```python
from build123d import *

# Parameters (mm, degrees)
SKETCH1_W              = 55.88
SKETCH1_H              = 63.5
EXTRUDE1_DEPTH         = 25.4
EXTRUDE1_DEPTH_BACK    = 25.4
EXTRUDE2_DEPTH         = 51.8
FILLET1_R              = 11.1125
F_10_CLEARANCE_HOLE1_D = 5.6134
LPATTERN1_COUNT        = 2
LPATTERN1_PITCH        = 15.24
SKETCH9_W              = 15.24
SKETCH9_H              = 37.338
EXTRUDE3_DEPTH         = 51.8
FILLET2_R              = 4.7625
EXTRUDE5_DEPTH         = 13.7
LPATTERN2_COUNT        = 2
LPATTERN2_PITCH        = 25.4
CHAMFER1_SIZE          = 2.54


with BuildPart() as part:
    # Sketch1 → Extrude1 (new body, two sides)
    with BuildSketch(Plane.XY) as extrude1_sk:
        Rectangle(SKETCH1_W, SKETCH1_H)
    extrude(amount=EXTRUDE1_DEPTH)
    extrude(extrude1_sk.sketch, amount=-EXTRUDE1_DEPTH_BACK)

    # Sketch2 → Extrude2 (cut, through all)
    with BuildSketch(Plane.XY.offset(25.4)):
        Polygon((-27.94, -31.75), (15.24, -31.75), (15.24, -16.51), (0, -16.51), (0, 31.75), (-27.94, 31.75), align=None)
    extrude(amount=-EXTRUDE2_DEPTH, mode=Mode.SUBTRACT)

    # Fillet1
    fillet1_edges = [part.edges().sort_by_distance(p)[0] for p in [
        (15.24, -16.51, 0),
    ]]
    fillet(fillet1_edges, radius=FILLET1_R)

    # 10 Clearance Hole1 (through all)
    with Locations(Plane(origin=(0, 31.75, 0), x_dir=(-1, 0, 0), z_dir=(0, 1, 0))):
        with Locations((-22.098, -7.62)):
            f_10_clearance_hole1 = Hole(F_10_CLEARANCE_HOLE1_D / 2)

    # LPattern1: 10 Clearance Hole1 ×2
    with Locations(*[(0, 0, i * LPATTERN1_PITCH) for i in range(1, LPATTERN1_COUNT)]):
        add(f_10_clearance_hole1, mode=Mode.SUBTRACT)

    # Sketch9 → Extrude3 (cut, through all)
    with BuildSketch(Plane.XY.offset(25.4)):
        with Locations((20.32, 13.081)):
            Rectangle(SKETCH9_W, SKETCH9_H)
    extrude(amount=-EXTRUDE3_DEPTH, mode=Mode.SUBTRACT)

    # Fillet2
    fillet2_edges = [part.edges().sort_by_distance(p)[0] for p in [
        (12.7, -5.588, 0),
    ]]
    fillet(fillet2_edges, radius=FILLET2_R)

    # Sketch11 → Extrude5 (cut, through all)
    with BuildSketch(Plane(origin=(12.7, 0, 0), x_dir=(0, 0, -1), z_dir=(1, 0, 0))):
        with BuildLine():
            Line((-9.3218, 20.32), (-9.3218, 12.7))
            ThreePointArc((-9.3218, 12.7), (-12.7, 9.3218), (-16.0782, 12.7))
            Line((-16.0782, 12.7), (-16.0782, 20.32))
            ThreePointArc((-16.0782, 20.32), (-12.7, 23.6982), (-9.3218, 20.32))
        make_face()
    extrude5 = extrude(amount=-EXTRUDE5_DEPTH, mode=Mode.SUBTRACT)

    # LPattern2: Extrude5 ×2
    with Locations(*[(0, 0, -i * LPATTERN2_PITCH) for i in range(1, LPATTERN2_COUNT)]):
        add(extrude5, mode=Mode.SUBTRACT)

    # Chamfer1
    chamfer1_edges = [part.edges().sort_by_distance(p)[0] for p in [
        (27.94, -18.669, -25.4),
        (27.94, -18.669, 25.4),
    ]]
    chamfer(chamfer1_edges, length=CHAMFER1_SIZE)


solid = part.part
```
Verification items for the finished model (mm, model axes). A direction names the side the tool comes from. Give positions to 0.01 mm unless a question says otherwise; leave off trailing zeros. Order: outer loops, then holes, each group sorted by start corner. A loop starts at its lowest first (then second) coordinate and runs counter-clockwise, first axis right, second up. Notation, with made-up numbers: M 18.5,53 L 26.5,53 A23 cw 26.5,85 Z; hole C -9.75,-36.5 d9. An arc over 180 degrees is marked long. Return JSON: item names as keys, results as strings. Group by question number.
1) Go/stop test with flat-tipped pins: pin 1 Ø9 at (x, z) = (22.098, 7.62) entering from +Y; pin 2 Ø1 at (x, z) = (7.5, 14.5) entering from -Y; pin 3 Ø11.5 at (x, z) = (22, 5) entering from +Y. Record where each tip stops, or that it passes through.
2) Section check A-A on y = 17. Record the cut outline in (x, z), and give its area (3 significant figures).
3) Access from +Z, -Z, +X, -X, +Y, -Y to the whole of each face (thin tool, end or side, straight path). Record for faces 4 (the face through (23, -5.588, 0)), 5 (the face through (6, 17, 9.322)), 6 (the face through (10, 0, -25.4)), 7 (the face through (2, -16.51, 0)).
4) Section check D-D on x = 8.5. Record the cut outline in (y, z).
5) Scan lines: line 1 (Z direction, x = 22.25, y = -23.5); line 2 (Z direction, x = 3.75, y = 18); line 3 (Y direction, x = 17.5, z = 17.5). Record each from-to range of solid material in increasing order.
6) Section check C-C on x = 20.75. Record the cut outline in (y, z), and give its area (3 significant figures).
7) Mould release check, pull along X, two halves, no side actions. Record for faces 1 (the face through (19.294, -18.852, -7.497)), 2 (the face through (6, 16, -9.322)), 3 (the face through (12.7, 15, 0)): pulls with the +X half, pulls with the -X half, needs draft (parallel to the pull), parting line crosses it, or undercut.
Answer block:
{
 "1": {"pin 1": "stops at y = -5.59", "pin 2": "stops at y = -17.21", "pin 3": "stops at y = -5.43"},
 "2": {"outline": "M 0,-25.4 L 12.7,-25.4 L 12.7,-16.08 L 0,-16.08 Z; M 0,-9.32 L 12.7,-9.32 L 12.7,9.32 L 0,9.32 Z; M 0,16.08 L 12.7,16.08 L 12.7,25.4 L 0,25.4 Z", "area": "474 mm^2"},
 "3": {"face 4": "+Z, -Z, +X, +Y", "face 5": "+X, -X", "face 6": "-Z, +X, -X, +Y, -Y", "face 7": "+Z, -Z, -X, -Y"},
 "4": {"outline": "M -17.41,-25.4 L 31.75,-25.4 L 31.75,25.4 L -17.41,25.4 Z; hole M 12.7,-16.08 L 20.32,-16.08 A3.38 ccw 20.32,-9.32 L 12.7,-9.32 A3.38 ccw Z; hole M 12.7,9.32 L 20.32,9.32 A3.38 ccw 20.32,16.08 L 12.7,16.08 A3.38 ccw Z"},
 "5": {"line 1": "z = -25.4 to -10.42, -4.82 to 4.82, 10.42 to 25.4", "line 2": "z = -25.4 to -16.08, -9.32 to 9.32, 16.08 to 25.4", "line 3": "y = -31.75 to -5.59"},
 "6": {"outline": "M -31.75,-25.4 L -5.59,-25.4 L -5.59,-10.08 L -31.75,-10.08 Z; M -31.75,-5.16 L -5.59,-5.16 L -5.59,5.16 L -31.75,5.16 Z; M -31.75,10.08 L -5.59,10.08 L -5.59,25.4 L -31.75,25.4 Z", "area": "1,070 mm^2"},
 "7": {"face 1": "undercut", "face 2": "needs draft", "face 3": "pulls with the +X half"}
}
